Geometry check sheet. Reference: the model listing, model coordinates, mm. A direction names the side the tool comes from. Coordinates: 2 decimals unless noted, no trailing zeros. Loops run counter-clockwise (first coordinate to the right, second up) from the corner with the lowest first, then second, coordinate; pieces in that order, holes last.
from build123d import *

# Parameters (mm, degrees)
F1_DEPTH = 8
F2_W     = 10.732
F2_H     = 6
F3_DEPTH = 25
F4_R     = 0.386274
F6_DEPTH = 8


with BuildPart() as f1:
    # F0 (on Top) → F1 (new body)
    with BuildSketch(Plane.XY):
        Polygon((11.366, 4), (-11.366, 4), (-11.366, 0), (-19.866, 0), (-19.866, -2.5), (-11.366, -2.5), (-11.366, -4), (-7.366, -4), (-7.366, 1.08), (7.366, 1.08), (7.366, -4), (11.366, -4), (11.366, -2.5), (19.866, -2.5), (19.866, 0), (11.366, 0), align=None)
    extrude(amount=F1_DEPTH)

    # F2 (on face) → F3 (cut)
    with BuildSketch(Plane.XZ.offset(-1.08)):
        with Locations((0, 4)):
            Rectangle(F2_W, F2_H)
    extrude(amount=-F3_DEPTH, mode=Mode.SUBTRACT)

    # F4
    f4_edges = [f1.edges().sort_by_distance(p)[0] for p in [
        (-5.366, 2.54, 1),
        (-5.366, 2.54, 7),
        (5.366, 2.54, 7),
        (5.366, 2.54, 1),
    ]]
    fillet(f4_edges, radius=F4_R)

    # F5 (on face) → F6 (join)
    with BuildSketch(Plane.XY.offset(8)):
        Polygon((19.866, 0), (11.366, 4), (11.366, 0), align=None)
        Polygon((-11.366, 0), (-11.366, 4), (-19.866, 0), align=None)
    extrude(amount=-F6_DEPTH)


solid = f1.part
1) Section check A-A on z = 2.5. Record the cut outline in (x, y).
Data:
outline: (-19.87, -2.5) - (-11.37, -2.5) - (-11.37, -4) - (-7.37, -4) - (-7.37, 1.08) - (-5.37, 1.08) - (-5.37, 4) - (-11.37, 4) - (-19.87, 0) - close; (5.37, 1.08) - (7.37, 1.08) - (7.37, -4) - (11.37, -4) - (11.37, -2.5) - (19.87, -2.5) - (19.87, 0) - (11.37, 4) - (5.37, 4) - close
2) Mould release check, pull along Z, two halves, no side actions. Record for faces 1 (the flat face through (0, 2, 0)), 2 (the flat face through (-7.366, -1, 4)), 3 (the flat face through (0, 3, 7)): +Z half, -Z half, draft (parallel to the pull), parting line (faces both ways), or undercut.
Data:
face 1: -Z half
face 2: draft
face 3: undercut
3) Depth check by flat-ended pin: pin 1 (2 mm diameter, centred on x = 15, z = 2.5, fed in from -Y); pin 2 (3 mm diameter, centred on y = 3, z = 3, fed in from -X); pin 3 (0.9 mm diameter, centred on y = 2, z = 5, fed in from +X). Enter the tip coordinate at first touch or a pass-through.
Data:
pin 1: stops at y = -2.5
pin 2: stops at x = -16.68
pin 3: stops at x = 16.57
4) Access from +Z, -Z, +X, -X, +Y, -Y to the whole of each face (thin tool, end or side, straight path). Record for faces 4 (the flat face through (-0.1, 1.08, 7.5)), 5 (the flat face through (16, -2.5, 4)), 6 (the flat face through (5.366, 3, 4)), 7 (the flat face through (15.68, 1.97, 4.06)), 8 (the flat face through (-11.366, -3, 4)).
Data:
face 4: +Z, -Z, -Y
face 5: +Z, -Z, +X, -Y
face 6: +Y, -Y
face 7: +Z, -Z, +X, +Y
face 8: +Z, -Z, -X, -Y
5) Section check B-B on x = 1.5. Record the cut outline in (y, z).
Data:
outline: (1.08, 0) - (4, 0) - (4, 1) - (1.08, 1) - close; (1.08, 7) - (4, 7) - (4, 8) - (1.08, 8) - close
6) Material ranges on probe 1 along Z at (x, y) = (5, 2.75); probe 2 along X at (y, z) = (-2.75, 1); probe 3 along Y at (x, z) = (-1, 7.75), recorded low to high.
Data:
probe 1: z = 0 to 1, 7 to 8
probe 2: x = -11.37 to -7.37, 7.37 to 11.37
probe 3: y = 1.08 to 4
7) Section check C-C on y = 2.5. Record the cut outline in (x, z).
Data:
outline: (-14.55, 0) - (14.55, 0) - (14.55, 8) - (-14.55, 8) - close; hole (-5.37, 1.39) arc R0.39 ccw to (-4.98, 1) - (4.98, 1) arc R0.39 ccw to (5.37, 1.39) - (5.37, 6.61) arc R0.39 ccw to (4.98, 7) - (-4.98, 7) arc R0.39 ccw to (-5.37, 6.61) - close
8) Section check D-D on z = 7.5. Record the cut outline in (x, y).
Data:
outline: (-19.87, -2.5) - (-11.37, -2.5) - (-11.37, -4) - (-7.37, -4) - (-7.37, 1.08) - (7.37, 1.08) - (7.37, -4) - (11.37, -4) - (11.37, -2.5) - (19.87, -2.5) - (19.87, 0) - (11.37, 4) - (-11.37, 4) - (-19.87, 0) - close
